Autodesk Inventor part; units mm, degrees
ref_plane "YZ Plane" through (0, 0, 0) normal (1, 0, 0) x (0, 1, 0)
ref_plane "XZ Plane" through (0, 0, 0) normal (0, 1, 0) x (-1, 0, 0)
ref_plane "XY Plane" through (0, 0, 0) normal (0, 0, 1) x (1, 0, 0)
sketch "Skizze1" plane through (0, 0, 0) normal (0, 0, 1) x (1, 0, 0)
  line L0 (-10.7, -35.5) -> (10.7, -35.5)
  line L1 (10.7, -35.5) -> (10.7, 35.5)
  line L2 (10.7, 35.5) -> (-10.7, 35.5)
  line L3 (-10.7, 35.5) -> (-10.7, -35.5)
  line L4 (-10.7, -35.5) -> (10.7, 35.5) construction
  line L5 (10.7, -35.5) -> (-10.7, 35.5) construction
  point P0 (0, 0)
  dimension "d0" = 21.4
  dimension "d1" = 71
extrude "Extrusion1" add sketch "Skizze1" along normal blind 2
sketch "Skizze2" plane through (0, 0, 2) normal (0, 0, 1) x (1, 0, 0)
  line L0 (10.7, 35.5) -> (-10.7, 35.5)
  line L1 (0, 35.5) -> (0, 32.4568) construction
  line L2 (-3.3034, 0) -> (2.2681, 0) construction
  line L3 (-10.7, 35.5) -> (-10.7, -35.5) construction
  circle A0 centre (8.08, 23.5) radius 1.5
  circle A1 centre (-8.08, -9.2) radius 1.5
  line L4 (9.58, 23.5) -> (10.7, 23.5)
  line L5 (10.7, -35.5) -> (10.7, 35.5)
  line L6 (-9.58, -9.2) -> (-10.7, -9.2)
  point P0 (0, 0)
  point P1 (10.14, 23.5)
  point P2 (-10.14, -9.2)
  dimension "d18" = 3
  dimension "d19" = 3
  dimension "d21" = 1.12
  dimension "d22" = 1.12
  dimension "d23" = 32.7
  dimension "d24" = 12
extrude "Extrusion2" cut sketch "Skizze2" against normal blind 4
sketch "Skizze3" plane through (0, 0, 0) normal (0, 0, -1) x (-1, 0, 0)
  line L0 (10.7, 35.5) -> (10.7, -35.5)
  line L1 (-10.7, -25.5) -> (10.7, -25.5)
  line L2 (10.7, -25.5) -> (10.7, 15.5)
  line L3 (10.7, 15.5) -> (-10.7, 15.5)
  line L4 (-10.7, 15.5) -> (-10.7, -25.5)
  line L5 (-10.7, -25.5) -> (10.7, 15.5) construction
  line L6 (10.7, -25.5) -> (-10.7, 15.5) construction
  line L7 (10.7, -35.5) -> (-10.7, -35.5)
  line L8 (-10.7, -35.5) -> (-10.7, 35.5)
  point P0 (0, -5)
  point P1 (10.7, -25.5)
  dimension "d9" = 41
  dimension "d17" = 10
extrude "Extrusion3" add sketch "Skizze3" along normal blind 13 contours L0 L1 L4 L3
sketch "Skizze4" plane through (-10.7, -35.5, 2) normal (-1, 0, 0) x (0, 0, 1)
  line L0 (-2, 10) -> (-15, 10)
  line L1 (-12.32, 10) -> (-2, 10)
  line L2 (-2, 10) -> (-2, 11.25)
  line L3 (-2, 11.25) -> (-12.32, 11.25)
  line L4 (-12.32, 11.25) -> (-12.32, 10)
  line L5 (-15, 10) -> (-15, 51)
  line L6 (-4.404, 30.5) -> (2.981, 30.5) construction
  line L7 (-2, 51) -> (-15, 51)
  line L8 (-2, 51) -> (-2, 49.75)
  line L9 (-2, 49.75) -> (-12.32, 49.75)
  line L10 (-12.32, 49.75) -> (-12.32, 51)
  line L11 (-2, 10) -> (-12.32, 10)
  point P0 (-2, 35.5)
  point P1 (-12.32, 10.625)
  dimension "d12" = 2.68
  dimension "d13" = 1.25
extrude "Extrusion4" cut sketch "Skizze4" against normal through all
fillet "Rundung1" radius 1 6 edges at (-10.7, -35.5, 1) (10.7, -35.5, 1) (10.7, 35.5, 1) (-10.7, 35.5, 1) (0, 15.5, -13) (0, -25.5, -13)
sketch "Skizze5" plane through (-10.7, -24.25, -10.32) normal (-1, 0, 0) x (0, 0, 1)
  line L0 (12.32, 16.55) -> (12.32, 13.55)
  line L1 (10.32, 13.55) -> (10.32, 16.55)
  line L2 (10.32, 13.55) -> (10.32, 16.55)
  line L3 (12.32, 16.55) -> (12.32, 13.55)
  circle A0 centre (8.82, 15.05) radius 1.5
  point P0 (10.32, 24.25)
  point P1 (10.32, 15.05)
  dimension "d25" = 3
loft "Erhebung2" cut profiles "Skizze5" section 2 edges at (-9.58, -9.2, 0)
properties part number "Relais_Platte_3D-Druck"
Build history of the part. All positions in model axes, mm. A direction names the side the tool comes from. Coordinates: 2 decimals unless noted, no trailing zeros. Order: outer loops, then holes, each group sorted by start corner. A loop starts at its lowest first (then second) coordinate and runs counter-clockwise, first axis right, second up.
Item 1: Saw through at B-B on y = 23.5. List the corners of the cut face in (x, z).
Filled in:
outline: (-10.7, 0) - (6.58, 0) - (6.58, 2) - (-10.7, 2) - close; (9.58, 0) - (10.7, 0) - (10.7, 2) - (9.58, 2) - close
Item 2: Saw through at C-C on x = 3.25. List the corners of the cut face in (y, z), then the cut area to 3 significant figures.
Filled in:
outline: (-35.5, 0) - (-24.25, 0) - (-24.25, -10.32) - (-25.5, -10.32) - (-25.5, -12) arc R1 ccw to (-24.5, -13) - (14.5, -13) arc R1 ccw to (15.5, -12) - (15.5, -10.32) - (14.25, -10.32) - (14.25, 0) - (35.5, 0) - (35.5, 2) - (-35.5, 2) - close
area: 649 mm2
Item 3: Tool access for faces 4 (the flat face through (0, 14.25, -5)), 5 (the flat face through (0, -25.5, -11)), 6 (the flat face through (0, 15.5, -11)): list every direction of +Z, -Z, +X, -X, +Y, -Y with a clear straight run to the whole face (end or side of a thin tool).
Filled in:
face 4: +X, -X, +Y
face 5: -Z, +X, -X, -Y
face 6: -Z, +X, -X, +Y
Item 4: Drill centre lines: L1, parallel to X at y = -9.2, z = 0.85; L2, parallel to Z at x = 5.75, y = 14.5; L3, parallel to Y at x = 8.08, z = 1.6. Where is each one in solid material? Low to high.
Filled in:
L1: x = -10.7 to -9.58, -6.58 to 10.7
L2: z = -13 to -10.32, 0 to 2
L3: y = -35.5 to 22, 25 to 35.5
Item 5: Saw through at D-D on z = -9. List the corners of the cut face in (x, y), then the cut area to 3 significant figures.
Filled in:
outline: (-10.7, -24.25) - (10.7, -24.25) - (10.7, 14.25) - (-10.7, 14.25) - close
area: 824 mm2
Item 6: Drop flat-ended pins along their axis: pin 1 Ø5 at (x, z) = (-5, -5.5) entering from +Y; pin 2 Ø5 at (x, y) = (8.08, 23.5) entering from -Z; pin 3 Ø1.8 at (x, z) = (2.5, -11.5) entering from +Y. Give the stop position or say it passes through.
Filled in:
pin 1: stops at y = 14.25
pin 2: stops at z = 0
pin 3: stops at y = 15.5
Item 7: Saw through at A-A on x = 8.08. List the corners of the cut face in (y, z).
Filled in:
outline: (-35.5, 0) - (-24.25, 0) - (-24.25, -10.32) - (-25.5, -10.32) - (-25.5, -12) arc R1 ccw to (-24.5, -13) - (14.5, -13) arc R1 ccw to (15.5, -12) - (15.5, -10.32) - (14.25, -10.32) - (14.25, 0) - (22, 0) - (22, 2) - (-35.5, 2) - close; (25, 0) - (35.5, 0) - (35.5, 2) - (25, 2) - close
Item 8: Mould opens along X. For faces 1 (the flat face through (0, -5, -13)), 2 (the flat face through (-10.7, -7, -5)), 3 (the cylindrical face through (7.885, 24.987, 1.014)) say: released by +X, released by -X, zero draft, split by the parting line, or undercut.
Filled in:
face 1: zero draft
face 2: released by -X
face 3: undercut
